Model file for the job. Use its own axes, mm. A direction names the side the tool comes from. Round coordinates to 2 decimals unless told otherwise and drop trailing zeros. Write each loop counter-clockwise with the first axis right and the second up, starting at its lowest first coordinate (ties: lowest second). Pieces come first, ordered by that corner, then holes.
```python
from build123d import *

# Parameters (mm, degrees)
F0_W     = 35.56
F0_H     = 35.56
F1_DEPTH = 5.08
F2_W     = 19.812
F2_H     = 4.572
F3_DEPTH = 2.54
F4_W     = 19.812
F4_H     = 4.572
F5_DEPTH = 2.54
F6_W     = 20.32
F6_H     = 5.08
F7_DEPTH = 2.54
F8_W     = 20.32
F8_H     = 5.08
F9_DEPTH = 2.54


with BuildPart() as f1:
    # F0 (on Top) → F1 (new body, symmetric)
    with BuildSketch(Plane.XY):
        Rectangle(F0_W, F0_H)
        Polygon((-1.5241102431, -2.7450520833), (-1.5241102431, -12.7), (-6.7771918403, -12.7), (-6.7771918403, 12.4850260417), (7.6591362847, 12.4850260417), (7.6591362847, 8.1083767361), (-1.5241102431, 8.1083767361), (-1.5241102431, 1.6150607639), (7.0197265625, 1.6150607639), (7.0197265625, -2.7450520833), align=None, mode=Mode.SUBTRACT)
    extrude(amount=F1_DEPTH, both=True)

    # F2 (on face) → F3 (join)
    with BuildSketch(Plane(origin=(0, 17.78, 0), x_dir=(-1, 0, 0), z_dir=(0, 1, 0))):
        Rectangle(F2_W, F2_H)
    extrude(amount=F3_DEPTH)

    # F4 (on face) → F5 (join)
    with BuildSketch(Plane(origin=(-17.78, 0, 0), x_dir=(0, -1, 0), z_dir=(-1, 0, 0))):
        Rectangle(F4_W, F4_H)
    extrude(amount=F5_DEPTH)

    # F6 (on face) → F7 (cut)
    with BuildSketch(Plane.XZ.offset(17.78)):
        Rectangle(F6_W, F6_H)
    extrude(amount=-F7_DEPTH, mode=Mode.SUBTRACT)

    # F8 (on face) → F9 (cut)
    with BuildSketch(Plane.YZ.offset(17.78)):
        Rectangle(F8_W, F8_H)
    extrude(amount=-F9_DEPTH, mode=Mode.SUBTRACT)


solid = f1.part
```
1) Wall check: probe 1 along Y at (x, z) = (1, 2); probe 2 along Y at (x, z) = (2, 2.5); probe 3 along X at (y, z) = (1, 4). Give the ranges that are in metal, low to high.
2) Flat gauge pins, fed straight in: pin 1 Ø3 at (x, z) = (2, -0.5) entering from -Y; pin 2 Ø3 at (y, z) = (-6, -0.5) entering from +X; pin 3 Ø1.3 at (x, y) = (-18.5, -4.5) entering from -Z; pin 4 Ø1.5 at (x, z) = (9.5, 0) entering from -Y. Where does each tip first touch, or does it go through?
3) Cut at A-A on x = 6. List the corners of the cut face in (y, z), and give its area (3 significant figures).
4) Cut at B-B on z = -3. List the corners of the cut face in (x, y).
5) Pull direction Z, two halves, no side cores. Call faces 1 (the face through (0, -17.78, 3)), 2 (the face through (10.16, -17, 0)), 3 (the face through (0, -4, 5.08)): released by +Z, released by -Z, zero draft, split by the parting line, or undercut.
6) Which spindle directions (+Z, -Z, +X, -X, +Y, -Y) get a long thin tool onto all of the face, cutting with end or side? Do faces 4 (the face through (3, 8.108, 0)), 5 (the face through (17, 0, 2.54)), 6 (the face through (0, -17, 2.54)), 7 (the face through (9.906, 19, 0)). Say none if no direction does.
7) Cut at C-C on y = 2.5. List the corners of the cut face in (x, z).
Result sheet:
1. probe 1: y = -15.24 to -2.75, 1.62 to 8.11, 12.49 to 20.32
1. probe 2: y = -15.24 to -2.75, 1.62 to 8.11, 12.49 to 17.78
1. probe 3: x = -17.78 to -6.78, 7.02 to 17.78
2. pin 1: stops at y = -15.24
2. pin 2: stops at x = 15.24
2. pin 3: stops at z = -2.29
2. pin 4: stops at y = -17.78
3. outline: (-17.78, -5.08) - (-2.75, -5.08) - (-2.75, 5.08) - (-17.78, 5.08) - (-17.78, 2.54) - (-15.24, 2.54) - (-15.24, -2.54) - (-17.78, -2.54) - close; (1.62, -5.08) - (8.11, -5.08) - (8.11, 5.08) - (1.62, 5.08) - close; (12.49, -5.08) - (17.78, -5.08) - (17.78, -2.29) - (20.32, -2.29) - (20.32, 2.29) - (17.78, 2.29) - (17.78, 5.08) - (12.49, 5.08) - close
3. area: 271 mm2
4. outline: (-17.78, -17.78) - (17.78, -17.78) - (17.78, 17.78) - (-17.78, 17.78) - close; hole (-6.78, -12.7) - (-1.52, -12.7) - (-1.52, -2.75) - (7.02, -2.75) - (7.02, 1.62) - (-1.52, 1.62) - (-1.52, 8.11) - (7.66, 8.11) - (7.66, 12.49) - (-6.78, 12.49) - close
5. face 1: zero draft
5. face 2: undercut
5. face 3: released by +Z
6. face 4: +Z, -Z
6. face 5: +X
6. face 6: -Y
6. face 7: +Z, -Z, +X, +Y
7. outline: (-20.32, -2.29) - (-17.78, -2.29) - (-17.78, -5.08) - (-6.78, -5.08) - (-6.78, 5.08) - (-17.78, 5.08) - (-17.78, 2.29) - (-20.32, 2.29) - close; (-1.52, -5.08) - (17.78, -5.08) - (17.78, -2.54) - (15.24, -2.54) - (15.24, 2.54) - (17.78, 2.54) - (17.78, 5.08) - (-1.52, 5.08) - close
